from build123d import *

# Parameters (mm, degrees)
SKETCH1_W           = 101.8286
SKETCH1_H           = 101.981
BOSS_EXTRUDE1_DEPTH = 10


with BuildPart() as part:
    # Sketch1 → Boss-Extrude1 (new body)
    with BuildSketch(Plane(origin=(0, 0, 0), x_dir=(1, 0, 0), z_dir=(0, 1, 0))):
        Rectangle(SKETCH1_W, SKETCH1_H)
    extrude(amount=BOSS_EXTRUDE1_DEPTH)

    # Cut-Sweep1: sweep along a path in Sketch2
    with BuildLine(Plane(origin=(0, 10, 0), x_dir=(1, 0, 0), z_dir=(0, 1, 0))) as cut_sweep1_path:
        Line((-42.493557128, -50.9905), (-42.493557128, 26.149650848))
        ThreePointArc((-42.493557128, 26.149650848), (-25.824807128, 42.818400848), (-9.156057128, 26.149650848))
        Line((-9.156057128, 26.149650848), (-9.156057128, -50.9905))
    # Sketch3 → Cut-Sweep1 (sweep, cut)
    with BuildSketch(Plane.XY.offset(50.9905)):
        with BuildLine():
            Line((-40.112307128, 10), (-44.874807128, 10))
            Line((-44.874807128, 10), (-44.874807128, 8.2))
            ThreePointArc((-44.874807128, 8.2), (-42.493557128, 5.81875), (-40.112307128, 8.2))
            Line((-40.112307128, 8.2), (-40.112307128, 10))
        make_face()
    sweep(path=cut_sweep1_path.line, mode=Mode.SUBTRACT)

    # Cut-Sweep2: sweep along a path in Sketch4
    with BuildLine(Plane(origin=(0, 10, 0), x_dir=(1, 0, 0), z_dir=(0, 1, 0))) as cut_sweep2_path:
        Line((10.2743, 50.9905), (10.2743, -50.9905))
    # Sketch5 → Cut-Sweep2 (sweep, cut)
    with BuildSketch(Plane.XY.offset(50.9905)):
        with BuildLine():
            Line((7.89305, 10), (12.65555, 10))
            Line((12.65555, 10), (12.65555, 7.9))
            ThreePointArc((12.65555, 7.9), (10.2743, 5.51875), (7.89305, 7.9))
            Line((7.89305, 7.9), (7.89305, 10))
        make_face()
        with BuildLine():
            Line((18.05305, 10), (22.81555, 10))
            Line((22.81555, 10), (22.81555, 8.1))
            ThreePointArc((22.81555, 8.1), (20.4343, 5.71875), (18.05305, 8.1))
            Line((18.05305, 8.1), (18.05305, 10))
        make_face()
        with BuildLine():
            Line((28.21305, 10), (32.97555, 10))
            Line((32.97555, 10), (32.97555, 8.3))
            ThreePointArc((32.97555, 8.3), (30.5943, 5.91875), (28.21305, 8.3))
            Line((28.21305, 8.3), (28.21305, 10))
        make_face()
        with BuildLine():
            Line((38.37305, 10), (43.13555, 10))
            Line((43.13555, 10), (43.13555, 8.5))
            ThreePointArc((43.13555, 8.5), (40.7543, 6.11875), (38.37305, 8.5))
            Line((38.37305, 8.5), (38.37305, 10))
        make_face()
        with BuildLine():
            Line((-2.26695, 10), (2.49555, 10))
            Line((2.49555, 10), (2.49555, 7.7))
            ThreePointArc((2.49555, 7.7), (0.1143, 5.31875), (-2.26695, 7.7))
            Line((-2.26695, 7.7), (-2.26695, 10))
        make_face()
    sweep(path=cut_sweep2_path.line, mode=Mode.SUBTRACT)


solid = part.part
CAD build for the part. Positions are in the model's coordinates, mm. A direction names the side the tool comes from. Round coordinates to 2 decimals unless told otherwise and drop trailing zeros. Loops run counter-clockwise (first coordinate to the right, second up) from the corner with the lowest first, then second, coordinate; pieces in that order, holes last.
(1) Cut at B-B (x = 10). Give the cut face in (y, z).
(2) Two-plate mould, pull along Z, no slides. Class faces 4 (the cylindrical face through (-26.139, 9.113, -40.434)), 5 (the flat face through (-2.267, 9, 1)), 6 (the flat face through (-1, 5, 50.99)), 7 (the cylindrical face through (-26.244, 9.087, -45.195)): +Z half, -Z half, draft (parallel to the pull), parting line (faces both ways), or undercut.
(3) Wall check: line 1 along Y through (x, z) = (40.5, -4); line 2 along Z through (x, y) = (-18, 8.75); line 3 along Y through (x, z) = (30.5, 41). Give the ranges that are in metal, low to high.
(4) Which spindle directions (+Z, -Z, +X, -X, +Y, -Y) get a long thin tool onto all of the face, cutting with end or side? Do faces 1 (the flat face through (-47, 10, -15)), 2 (the cylindrical face through (-42.44, 5.82, 11.88)), 3 (the flat face through (2.496, 9, 1)). Say none if no direction does.
Findings below:
1. outline: (0, -50.99) - (5.53, -50.99) - (5.53, 50.99) - (0, 50.99) - close
2. face 4: undercut
2. face 5: draft
2. face 6: +Z half
2. face 7: undercut
3. line 1: y = 0 to 6.13
3. line 2: z = -50.99 to -43.52, -38.1 to 50.99
3. line 3: y = 0 to 5.92
4. face 1: +Z, -Z, +X, -X, +Y
4. face 2: +Z, +Y
4. face 3: +Z, -Z, +Y
